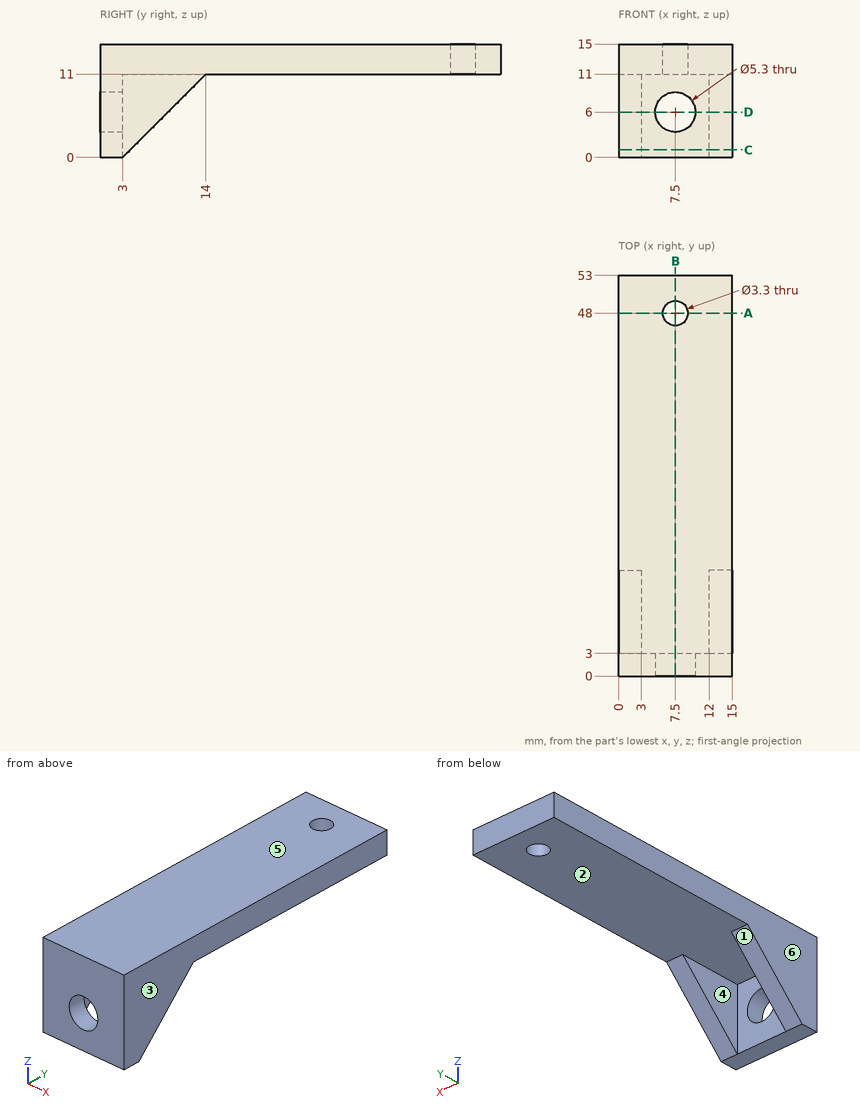
The drawing under review shows one solid part. Ordinate dimensions are in mm from its lowest x, y, z. A direction names the side the tool comes from. Round coordinates to 2 decimals unless told otherwise and drop trailing zeros. Loops run counter-clockwise (first coordinate to the right, second up) from the corner with the lowest first, then second, coordinate; pieces in that order, holes last. Notation, with made-up numbers: (51.25, -15.75) - (91.25, -15.75) arc R22 ccw to (91.25, 16.25) - close; hole circle Ø8 at (19.5, -9). An arc over 180 degrees is marked (long way). Use one line per item in the form item = value.
Item 1: Consider section B-B on x = 7.5. Write out the cut boundary in (y, z), then the cut area to 3 significant figures.
Answers:
outline = (0, 0) - (3, 0) - (3, 3.35) - (0, 3.35) - close; (0, 8.65) - (3, 8.65) - (3, 11) - (46.35, 11) - (46.35, 15) - (0, 15) - close; (49.65, 11) - (53, 11) - (53, 15) - (49.65, 15) - close
area = 216 mm^2
Item 2: Mouldability with a two-part tool opening along X and no side actions: class the marked faces 3, 4, 5 and 6 as +X half, -X half, draft (parallel to the pull), parting line (faces both ways), or undercut.
Answers:
face_3 = +X half
face_4 = undercut
face_5 = draft
face_6 = -X half
Item 3: Consider section D-D on z = 6. Write out the cut boundary in (x, y), then the cut area to 3 significant figures.
Answers:
outline = (0, 0) - (4.85, 0) - (4.85, 3) - (3, 3) - (3, 9) - (0, 9) - close; (10.15, 0) - (15, 0) - (15, 9) - (12, 9) - (12, 3) - (10.15, 3) - close
area = 65.1 mm^2
Item 4: Tool access review of the marked faces 1 and 2: name each direction out of +Z, -Z, +X, -X, +Y, -Y from which nothing blocks a thin tool from reaching the whole face with its end or side.
Answers:
face_1 = -Z, +X, -X, +Y
face_2 = -Z, +Y
Item 5: Consider section C-C on z = 1. Write out the cut boundary in (x, y), then the cut area to 3 significant figures.
Answers:
outline = (0, 0) - (15, 0) - (15, 4) - (12, 4) - (12, 3) - (3, 3) - (3, 4) - (0, 4) - close
area = 51.0 mm^2
Item 6: Consider section A-A on y = 48. Write out the cut boundary in (x, z), then the cut area to 3 significant figures.
Answers:
outline = (0, 11) - (5.85, 11) - (5.85, 15) - (0, 15) - close; (9.15, 11) - (15, 11) - (15, 15) - (9.15, 15) - close
area = 46.8 mm^2
Item 7: Clearance check with flat-ended pins moving along their axes: P1, Ø5, axis at x = 4.5, y = 6.5, coming from the -Z side; P2, Ø7.5, axis at x = 8.5, y = 34.5, coming from the -Z side; P3, Ø4, axis at x = 7.5, z = 6, coming from the +Y side; P4, Ø2, axis at x = 2.5, z = 7.5, coming from the +Y side. State where each tip first meets the part, or that it passes through.
Answers:
P1 = 1.5
P2 = 11
P3 = through
P4 = 11.5
Item 8: For line 1 (X direction, y = 0.9, z = 6); line 2 (Y direction, x = 11, z = 1.25); line 3 (Z direction, x = 5.25, y = 40.5), list the stretches that pass through material, from the lowest coordinate up.
Answers:
line_1 = 0 to 4.85, 10.15 to 15
line_2 = 0 to 3
line_3 = 11 to 15
